```python
from build123d import *

# Parameters (mm, degrees)
ESQUISSE16_R        = 1.5
BOSS_EXTRU_16_DEPTH = 3


with BuildPart() as part:
    # Esquisse16 → Boss.-Extru.16 (new body)
    with BuildSketch(Plane.XY):
        with BuildLine():
            Line((27.030251009, -10.651447746), (54.030251009, -10.651447746))
            ThreePointArc((54.030251009, -10.651447746), (56.151571352, -11.530127403), (57.030251009, -13.651447746))
            Line((57.030251009, -13.651447746), (57.030251009, -31.651447746))
            ThreePointArc((57.030251009, -31.651447746), (56.151571352, -33.77276809), (54.030251009, -34.651447746))
            Line((54.030251009, -34.651447746), (27.030251009, -34.651447746))
            ThreePointArc((27.030251009, -34.651447746), (24.908930665, -33.77276809), (24.030251009, -31.651447746))
            Line((24.030251009, -31.651447746), (24.030251009, -13.651447746))
            ThreePointArc((24.030251009, -13.651447746), (24.908930665, -11.530127403), (27.030251009, -10.651447746))
        make_face()
        with Locations((27.030251009, -13.651447746)):
            Circle(ESQUISSE16_R, mode=Mode.SUBTRACT)
        with Locations((54.030251009, -13.651447746)):
            Circle(ESQUISSE16_R, mode=Mode.SUBTRACT)
        with Locations((54.030251009, -31.651447746)):
            Circle(ESQUISSE16_R, mode=Mode.SUBTRACT)
        with Locations((27.030251009, -31.651447746)):
            Circle(ESQUISSE16_R, mode=Mode.SUBTRACT)
        Polygon((29.030251009, -28.651447746), (34.530251009, -28.651447746), (34.530251009, -31.651447746), (46.530251009, -31.651447746), (46.530251009, -28.651447746), (52.030251009, -28.651447746), (52.030251009, -25.151447746), (53.530251009, -25.151447746), (53.530251009, -20.151447746), (52.030251009, -20.151447746), (52.030251009, -16.651447746), (46.530251009, -16.651447746), (46.530251009, -13.651447746), (34.530251009, -13.651447746), (34.530251009, -16.651447746), (29.030251009, -16.651447746), (29.030251009, -20.151447746), (27.530251009, -20.151447746), (27.530251009, -25.151447746), (29.030251009, -25.151447746), align=None, mode=Mode.SUBTRACT)
    extrude(amount=BOSS_EXTRU_16_DEPTH)


solid = part.part
```
Input: part model. Units: mm. Frame: model coordinates. A direction names the side the tool comes from. Give positions to 0.01 mm unless a question says otherwise; leave off trailing zeros. Order: outer loops, then holes, each group sorted by start corner. A loop starts at its lowest first (then second) coordinate and runs counter-clockwise, first axis right, second up.
1. Cut plane B-B (z = 0.35). State how many separate pieces and enclosed holes the cut face has, and give its area (3 significant figures).
Computed:
separate pieces: 1
enclosed holes: 5
area: 393 mm2
2. Line query: probe 1 along Y at (x, z) = (27, 1.15); probe 2 along Y at (x, z) = (29, 2.5); probe 3 along Y at (x, z) = (39, 1.45). Output: solid intervals per line, ascending.
Computed:
probe 1: y = -34.65 to -33.15, -30.15 to -15.15, -12.15 to -10.65
probe 2: y = -34.65 to -25.15, -20.15 to -10.65
probe 3: y = -34.65 to -31.65, -13.65 to -10.65
3. Pin query (flat end, axial travel): pin 1 Ø5 at (x, y) = (50.5, -28) entering from -Z. Return the tip coordinate at first contact, or that it passes through.
Computed:
pin 1: stops at z = 0
4. Cut plane D-D (y = -14). Return loops of the section in (x, z).
Computed:
outline: (24.03, 0) - (25.57, 0) - (25.57, 3) - (24.03, 3) - close; (28.49, 0) - (34.53, 0) - (34.53, 3) - (28.49, 3) - close; (46.53, 0) - (52.57, 0) - (52.57, 3) - (46.53, 3) - close; (55.49, 0) - (57.03, 0) - (57.03, 3) - (55.49, 3) - close
5. Draft query along X for faces 1 (the face through (24.932, -33.796, 1.479)), 2 (the face through (40, -10.651, 1)), 3 (the face through (28, -20.151, 1)). Return one class per face: released by +X, released by -X, zero draft, split by the parting line, or undercut.
Computed:
face 1: released by -X
face 2: zero draft
face 3: undercut
6. Cut plane C-C (y = -24.75). Return loops of the section in (x, z).
Computed:
outline: (24.03, 0) - (27.53, 0) - (27.53, 3) - (24.03, 3) - close; (53.53, 0) - (57.03, 0) - (57.03, 3) - (53.53, 3) - close
7. Set-up query: faces 4 (the face through (24.03, -23, 1)), 5 (the face through (49, -16.651, 1)). Return all of +Z, -Z, +X, -X, +Y, -Y with unobstructed straight access to the full face (end or side cutting, diameter ignored); none if empty.
Computed:
face 4: +Z, -Z, -X, +Y, -Y
face 5: +Z, -Z
8. Cut plane A-A (x = 44.5). Return loops of the section in (y, z), and give its area (3 significant figures).
Computed:
outline: (-34.65, 0) - (-31.65, 0) - (-31.65, 3) - (-34.65, 3) - close; (-13.65, 0) - (-10.65, 0) - (-10.65, 3) - (-13.65, 3) - close
area: 18.0 mm2
